from build123d import *

# Parameters (mm, degrees)
EXTRUDE_1_DEPTH = 150


with BuildPart() as part:
    # Эскиз1 → Бобышка-Вытянуть1 (new body)
    with BuildSketch(Plane.XY):
        Polygon((2.598076211, 44.688021535), (-2.598076211, 44.688021535), (-37.401923789, 24.594010768), (-40, 20.094010768), (-40, -20.094010768), (-37.401923789, -24.594010768), (-2.598076211, -44.688021535), (2.598076211, -44.688021535), (37.401923789, -24.594010768), (40, -20.094010768), (40, 20.094010768), (37.401923789, 24.594010768), align=None)
        Polygon((-2.062177826, 42.688021535), (-35.937822174, 23.129909152), (-38, 19.558112383), (-38, -19.558112383), (-35.937822174, -23.129909152), (-2.062177826, -42.688021535), (2.062177826, -42.688021535), (35.937822174, -23.129909152), (38, -19.558112383), (38, 19.558112383), (35.937822174, 23.129909152), (2.062177826, 42.688021535), align=None, mode=Mode.SUBTRACT)
    extrude(amount=EXTRUDE_1_DEPTH)


solid = part.part
Part model, mm, in its own coordinate system. A direction names the side the tool comes from. Coordinates: 2 decimals unless noted, no trailing zeros. Order: outer loops, then holes, each group sorted by start corner. A loop starts at its lowest first (then second) coordinate and runs counter-clockwise, first axis right, second up.
(1) Probe L1, parallel to X at y = 17, z = 98; L2, parallel to Y at x = -17, z = 19.5; L3, parallel to Y at x = 18.5, z = 137. List the from-to ranges inside material, lowest first.
Check sheet entries:
L1: x = -40 to -38, 38 to 40
L2: y = -36.37 to -34.06, 34.06 to 36.37
L3: y = -35.51 to -33.2, 33.2 to 35.51
(2) Slice it at C-C, the plane x = 11. Write the cut outline in (y, z), and give its area (3 significant figures).
Check sheet entries:
outline: (-39.84, 0) - (-37.53, 0) - (-37.53, 150) - (-39.84, 150) - close; (37.53, 0) - (39.84, 0) - (39.84, 150) - (37.53, 150) - close
area: 693 mm2
(3) Tool access for faces 1 (the face through (0, -44.688, 74)), 2 (the face through (18.763, -33.046, 73.95)): list every direction of +Z, -Z, +X, -X, +Y, -Y with a clear straight run to the whole face (end or side of a thin tool).
Check sheet entries:
face 1: +Z, -Z, +X, -X, -Y
face 2: +Z, -Z
(4) Slice it at B-B, the plane z = 71. Write the cut outline in (x, y), and give its area (3 significant figures).
Check sheet entries:
outline: (-40, -20.09) - (-37.4, -24.59) - (-2.6, -44.69) - (2.6, -44.69) - (37.4, -24.59) - (40, -20.09) - (40, 20.09) - (37.4, 24.59) - (2.6, 44.69) - (-2.6, 44.69) - (-37.4, 24.59) - (-40, 20.09) - close; hole (-38, -19.56) - (-35.94, -23.13) - (-2.06, -42.69) - (2.06, -42.69) - (35.94, -23.13) - (38, -19.56) - (38, 19.56) - (35.94, 23.13) - (2.06, 42.69) - (-2.06, 42.69) - (-35.94, 23.13) - (-38, 19.56) - close
area: 532 mm2
(5) Slice it at A-A, the plane y = 18. Write the cut outline in (x, z).
Check sheet entries:
outline: (-40, 0) - (-38, 0) - (-38, 150) - (-40, 150) - close; (38, 0) - (40, 0) - (40, 150) - (38, 150) - close
(6) Pull direction X, two halves, no side cores. Call faces 3 (the face through (36.954, -21.369, 73.95)), 4 (the face through (19.76, -34.78, 73.95)), 5 (the face through (-20.244, -34.5, 73.95)): pulls with the +X half, pulls with the -X half, needs draft (parallel to the pull), parting line crosses it, or undercut.
Check sheet entries:
face 3: undercut
face 4: pulls with the +X half
face 5: pulls with the -X half
(7) Pin check, flat tips, straight feed: pin 1 Ø3 at (y, z) = (-35.5, 55) entering from -X; pin 2 Ø3 at (y, z) = (-23.5, 22.5) entering from +X. Stop position of each tip, or through.
Check sheet entries:
pin 1: stops at x = -21.11
pin 2: stops at x = 38.9
